```python
from build123d import *

# Parameters (mm, degrees)
BOSS_EXTRUDE1_DEPTH = 2
SKETCH2_W           = 1.100075991
SKETCH2_H           = 6.000695173
BOSS_EXTRUDE2_DEPTH = 1.5
SKETCH3_W           = 1.500075991
SKETCH3_H           = 6.400695173
BOSS_EXTRUDE3_DEPTH = 1
CHAMFER1_SIZE       = 0.2


with BuildPart() as part:
    # Sketch1 → Boss-Extrude1 (new body)
    with BuildSketch(Plane(origin=(0, 0, 0), x_dir=(-1, 0, 0), z_dir=(0, 0, -1))):
        Polygon((-262.955830275, 81.455427603), (-266.055906266, 81.455427603), (-266.055906266, 71.95473243), (-273.006316619, 71.95473243), (-296.80691239, 71.95473243), (-296.80691239, 81.455427603), (-299.906988381, 81.455427603), (-299.906988381, 69.95473243), (-262.955830275, 69.95473243), align=None)
    extrude(amount=BOSS_EXTRUDE1_DEPTH)

    # Sketch2 → Boss-Extrude2 (add)
    with BuildSketch(Plane.XY):
        with Locations((265.505868271, 78.455080017)):
            Rectangle(SKETCH2_W, SKETCH2_H)
        with Locations((297.356950385, 78.455080017)):
            Rectangle(SKETCH2_W, SKETCH2_H)
    extrude(amount=BOSS_EXTRUDE2_DEPTH)

    # Sketch3 → Boss-Extrude3 (add)
    with BuildSketch(Plane.XY.offset(1.5)):
        with Locations((265.305868271, 78.255080017)):
            Rectangle(SKETCH3_W, SKETCH3_H)
        with Locations((297.556950386, 78.255080017)):
            Rectangle(SKETCH3_W, SKETCH3_H)
    extrude(amount=BOSS_EXTRUDE3_DEPTH)

    # Chamfer1
    chamfer1_edges = [part.edges().sort_by_distance(p)[0] for p in [
        (264.555830275, 78.255080016, 1.5),
        (265.305868271, 75.05473243, 1.5),
        (297.556950386, 75.05473243, 1.5),
        (298.306988381, 78.255080016, 1.5),
    ]]
    chamfer(chamfer1_edges, length=CHAMFER1_SIZE)


solid = part.part
```
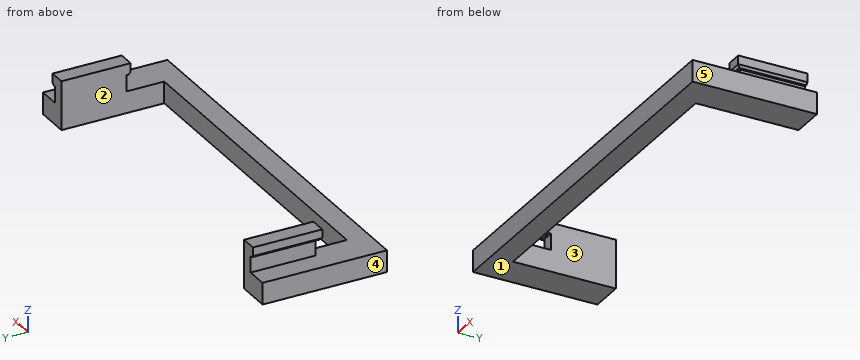
Geometry: final body of the model. Coordinates: model frame, mm. Face numbers are marked on the shaded views. A direction names the side the tool comes from. Give positions to 0.01 mm unless a question says otherwise; leave off trailing zeros. Write each loop counter-clockwise with the first axis right and the second up, starting at its lowest first coordinate (ties: lowest second). Pieces come first, ordered by that corner, then holes.
1. Reachability of the marked faces 1 and 2 from +Z, -Z, +X, -X, +Y, -Y: full face, straight path, thin tool, end or side. Return the list, or none.
2. Pin query (flat end, axial travel): P1, Ø0.9, axis at x = 298, z = 2, coming from the -Y side; P2, Ø0.9, axis at y = 79.5, z = 2, coming from the +X side; P3, Ø0.9, axis at y = 77, z = 2, coming from the -X side. Return the tip coordinate at first contact, or that it passes through.
3. Section query D-D, the plane x = 269. Return loops of the section in (y, z).
4. Line query: probe 1 along X at (y, z) = (72.25, -1.75); probe 2 along X at (y, z) = (78, 0.15); probe 3 along Z at (x, y) = (290, 71.75). Output: solid intervals per line, ascending.
5. Draft query along X for the marked faces 3, 4 and 5. Return one class per face: released by +X, released by -X, zero draft, split by the parting line, or undercut.
6. Section query B-B, the plane z = -1. Return loops of the section in (x, y).
7. Section query C-C, the plane z = 0.75. Return loops of the section in (x, y).
8. Section query A-A, the plane y = 76.75. Return loops of the section in (x, z).
Computed:
1. face 1: -Z, +X, -X, +Y, -Y
1. face 2: +Z, -Z, +Y
2. P1: stops at y = 75.05
2. P2: stops at x = 298.31
2. P3: stops at x = 264.56
3. outline: (69.95, -2) - (71.95, -2) - (71.95, 0) - (69.95, 0) - close
4. probe 1: x = 262.96 to 266.06, 296.81 to 299.91
4. probe 2: x = 264.96 to 266.06, 296.81 to 297.91
4. probe 3: z = -2 to 0
5. face 3: undercut
5. face 4: released by -X
5. face 5: released by +X
6. outline: (262.96, 69.95) - (299.91, 69.95) - (299.91, 81.46) - (296.81, 81.46) - (296.81, 71.95) - (266.06, 71.95) - (266.06, 81.46) - (262.96, 81.46) - close
7. outline: (264.96, 75.45) - (266.06, 75.45) - (266.06, 81.46) - (264.96, 81.46) - close; (296.81, 75.45) - (297.91, 75.45) - (297.91, 81.46) - (296.81, 81.46) - close
8. outline: (262.96, -2) - (266.06, -2) - (266.06, 2.5) - (264.56, 2.5) - (264.56, 1.7) - (264.76, 1.5) - (264.96, 1.5) - (264.96, 0) - (262.96, 0) - close; (296.81, -2) - (299.91, -2) - (299.91, 0) - (297.91, 0) - (297.91, 1.5) - (298.11, 1.5) - (298.31, 1.7) - (298.31, 2.5) - (296.81, 2.5) - close
